Model file for the job. Use its own axes, mm. A direction names the side the tool comes from. Give positions to 0.01 mm unless a question says otherwise; leave off trailing zeros. Write each loop counter-clockwise with the first axis right and the second up, starting at its lowest first coordinate (ties: lowest second). Pieces come first, ordered by that corner, then holes. Notation, with made-up numbers: (-13.5, 58) - (27.5, 58) arc R26 ccw to (27.5, 90) - close; hole circle Ø7 at (-11, 45). An arc over 180 degrees is marked (long way). One line per item, written item: value. Start each with the question number.
(1) Cut at A-A, the plane y = 0. List the corners of the cut face in (x, z).
(2) Cut at D-D, the plane x = -4. List the corners of the cut face in (y, z), and give its area (3 significant figures).
(3) Cut at B-B, the plane x = 0. List the corners of the cut face in (y, z).
(4) Cut at C-C, the plane y = -6.5. List the corners of the cut face in (x, z), and give its area (3 significant figures).
(5) Probe L1, parallel to Z at x = 0, y = -4; L2, parallel to X at y = 0, z = 10.7; L3, parallel to Y at x = 0, z = 26. List the from-to ranges inside material, lowest first.
(6) Mould opens along Y. For faces 1 (the face through (-1.62, 7.28, 32.99)), 2 (the face through (0, 4, 11.817)), 3 (the face through (-1.1, 5.5, 57.466)) say: pulls with the +Y half, pulls with the -Y half, needs draft (parallel to the pull), parting line crosses it, or undercut.
(7) 3-axis set-ups, long thin cutter, end or side, ignore diameter. For faces 4 (the face through (-0.711, -5.412, 9.789)), 5 (the face through (-0.711, -5.412, 59.494)), 6 (the face through (-1.5, -5.26, 51.23)), 7 (the face through (1.1, 5.5, 7.817)): which of +Z, -Z, +X, -X, +Y, -Y reach the whole face in a straight line?
(8) Drop flat-ended pins along their axis: P1, Ø3.5, axis at x = 0, y = -2.5, coming from the -Z side; P2, Ø2.5, axis at x = 0, z = 17.55, coming from the -Y side; P3, Ø6, axis at x = 0, y = 0, coming from the -Z side; P4, Ø1, axis at y = 6, z = 56, coming from the -X side. Give the stop position or say it passes through.
from build123d import *

# Parameters (mm, degrees)
F3_D     = 3
F3_DEPTH = 7.4598419297


with BuildPart() as f1:
    # F0 (on Front) → F1 (revolve)
    with BuildSketch(Plane.XZ):
        Polygon((3.4588419297, 61.4661982319), (3.4588419297, 11.8165865856), (5.4588419297, 11.8165865856), (5.4588419297, 7.8165865856), (7.4588419297, 7.8165865856), (7.4588419297, 57.4661982319), (5.4588419297, 57.4661982319), (5.4588419297, 61.4661982319), align=None)
    revolve(axis=Axis((0, 0, 33.0960974097), (0, 0, -1)))

    # F3 (through all, one way)
    with BuildSketch(Plane(origin=(0, 0, 0), x_dir=(1, 0, 0), z_dir=(0, 1, 0))):
        with Locations((0, -51.2947626412), (0, -35.1628810167), (0, -17.5476111472)):
            Circle(F3_D / 2)
    extrude(amount=-F3_DEPTH, mode=Mode.SUBTRACT)


solid = f1.part
Answers follow:
1. outline: (-7.46, 7.82) - (-5.46, 7.82) - (-5.46, 11.82) - (-3.46, 11.82) - (-3.46, 61.47) - (-5.46, 61.47) - (-5.46, 57.47) - (-7.46, 57.47) - close; (3.46, 11.82) - (5.46, 11.82) - (5.46, 7.82) - (7.46, 7.82) - (7.46, 57.47) - (5.46, 57.47) - (5.46, 61.47) - (3.46, 61.47) - close
2. outline: (-6.3, 7.82) - (-3.71, 7.82) - (-3.71, 11.82) - (3.71, 11.82) - (3.71, 7.82) - (6.3, 7.82) - (6.3, 57.47) - (3.71, 57.47) - (3.71, 61.47) - (-3.71, 61.47) - (-3.71, 57.47) - (-6.3, 57.47) - close
2. area: 625 mm²
3. outline: (-7.46, 7.82) - (-5.46, 7.82) - (-5.46, 11.82) - (-3.46, 11.82) - (-3.46, 16.05) - (-7.46, 16.05) - close; (-7.46, 19.05) - (-3.46, 19.05) - (-3.46, 33.66) - (-7.46, 33.66) - close; (-7.46, 36.66) - (-3.46, 36.66) - (-3.46, 49.79) - (-7.46, 49.79) - close; (-7.46, 52.79) - (-3.46, 52.79) - (-3.46, 61.47) - (-5.46, 61.47) - (-5.46, 57.47) - (-7.46, 57.47) - close; (3.46, 11.82) - (5.46, 11.82) - (5.46, 7.82) - (7.46, 7.82) - (7.46, 57.47) - (5.46, 57.47) - (5.46, 61.47) - (3.46, 61.47) - close
4. outline: (-3.66, 7.82) - (3.66, 7.82) - (3.66, 57.47) - (-3.66, 57.47) - close; hole circle Ø3 at (0, 17.55); hole circle Ø3 at (0, 35.16); hole circle Ø3 at (0, 51.29)
4. area: 342 mm²
5. L1: z = 11.82 to 16.05, 19.05 to 33.66, 36.66 to 49.79, 52.79 to 61.47
5. L2: x = -7.46 to -5.46, 5.46 to 7.46
5. L3: y = -7.46 to -3.46, 3.46 to 7.46
6. face 1: parting line crosses it
6. face 2: undercut
6. face 3: needs draft
7. face 4: -Z
7. face 5: +Z
7. face 6: -Y
7. face 7: -Z, +X, -X, +Y, -Y
8. P1: stops at z = 11.82
8. P2: stops at y = 3.23
8. P3: passes through
8. P4: stops at x = -5.04
